Source: CAD feature listing. Evaluate the final solid. Frame: model axes, mm. A direction names the side the tool comes from. Round coordinates to 2 decimals unless told otherwise and drop trailing zeros. Loops run counter-clockwise (first coordinate to the right, second up) from the corner with the lowest first, then second, coordinate; pieces in that order, holes last. Notation, with made-up numbers: M 78.5,54.5 L 109.5,54.5 A25 ccw 109.5,83.5 Z; hole C 10,62 d3. An arc over 180 degrees is marked long. Write each question's results on one line, items separated by ' | '. Start each with the question number.
1. Section B-B on x = 0. Output: boundary loops of the cut face in (y, z).
2. Section D-D on y = 11.75. Output: boundary loops of the cut face in (x, z).
3. Draft query along Y for faces 1 (the flat face through (0, 18, 2.5)), 2 (the flat face through (-3, 12.5, 1)), 3 (the cylindrical face through (-0.26, 20.67, 1.23)). Return one class per face: released by +Y, released by -Y, zero draft, split by the parting line, or undercut.
4. Set-up query: faces 4 (the cylindrical face through (1.88, 6.16, 5.96)), 5 (the cylindrical face through (-2.662, 15.208, 1.384)), 6 (the flat face through (0, 14.5, -1)). Return all of +Z, -Z, +X, -X, +Y, -Y with unobstructed straight access to the full face (end or side cutting, diameter ignored); none if empty.
5. Contact query for flat-ended pins moving along their axis: pin 1 Ø2 at (x, z) = (-3.5, -2.5) entering from +Y; pin 2 Ø1.4 at (x, y) = (0, 19.5) entering from +Z; pin 3 Ø1.5 at (x, z) = (0.5, -2) entering from +Y; pin 4 Ø3 at (y, z) = (7, -2) entering from +X. Output: stop coordinate, or through.
6. Section A-A on y = 19.5. Output: boundary loops of the cut face in (x, z), and give its area (3 significant figures).
7. Section C-C on z = 2.75. Output: boundary loops of the cut face in (x, y), and give its area (3 significant figures).
8. Ray query, line 1 (Y direction, x = 0, z = 1.1); line 2 (Z direction, x = 0.25, y = 17); line 3 (Y direction, x = 5.75, z = -1.5). Return the intervals inside material, ascending.
from build123d import *

# Parameters (mm, degrees)
F2_W          = 9.5753744735
F2_H          = 5.0194775218
F2_H_2        = 2.1959905885
F3_DEPTH      = 6.251
F3_DEPTH_BACK = 6.251
F4_R          = 1.2
F5_DEPTH      = 6.251


with BuildPart() as f1:
    # F0 (on Right) → F1 (revolve)
    with BuildSketch(Plane.YZ):
        Polygon((0, 6.25), (0, 0), (22.5, 0), (22.5, 3), (12.5, 3), (12.5, 6.25), align=None)
    revolve(axis=Axis((0, 13.297872428, 0), (0, 1, 0)))

    # F2 (on Right) → F3 (cut, two sides)
    with BuildSketch(Plane.YZ) as f3_sk:
        with Locations((19.2876872367, -2.5097387609)):
            Rectangle(F2_W, F2_H)
        with Locations((19.2876872367, 3.5979952943)):
            Rectangle(F2_W, F2_H_2)
    extrude(amount=-F3_DEPTH, mode=Mode.SUBTRACT)
    extrude(f3_sk.sketch, amount=F3_DEPTH_BACK, mode=Mode.SUBTRACT)

    # F4 (on face) → F5 (cut, through all)
    with BuildSketch(Plane(origin=(0, 0, 0), x_dir=(1, 0, 0), z_dir=(0, 0, -1))):
        with Locations((0, -19.5)):
            Circle(F4_R)
    extrude(amount=-F5_DEPTH, mode=Mode.SUBTRACT)


solid = f1.part
Taken from the geometry:
1) outline: M 0,-6.25 L 12.5,-6.25 L 12.5,-3 L 14.5,-3 L 14.5,0 L 18.3,0 L 18.3,2.5 L 14.5,2.5 L 14.5,3 L 12.5,3 L 12.5,6.25 L 0,6.25 Z; M 20.7,0 L 22.5,0 L 22.5,2.5 L 20.7,2.5 Z
2) outline: C 0,0 d12.5
3) face 1: zero draft | face 2: released by +Y | face 3: undercut
4) face 4: +Y, -Y | face 5: +Y | face 6: -Z, +X, -X, +Y
5) pin 1: y = 12.5 | pin 2: through | pin 3: y = 14.5 | pin 4: x = 6.23
6) outline: M -3,0 L -1.2,0 L -1.2,2.5 L -1.66,2.5 A3 ccw Z; M 1.2,0 L 3,0 A3 ccw 1.66,2.5 L 1.2,2.5 Z | area: 7.01 mm^2
7) outline: M -5.61,0 L 5.61,0 L 5.61,12.5 L 1.2,12.5 L 1.2,14.5 L -1.2,14.5 L -1.2,12.5 L -5.61,12.5 Z | area: 145 mm^2
8) line 1: 0 to 18.3, 20.7 to 22.5 | line 2: 0 to 2.5 | line 3: 0 to 12.5
